```python
from build123d import *

# Parameters (mm, degrees)
SKETCH1_W           = 70
SKETCH1_H           = 132
BOSS_EXTRUDE1_DEPTH = 3
SKETCH2_R           = 1.6
SKETCH2_R_2         = 8
CUT_EXTRUDE1_DEPTH  = 75.76630257
CUT_EXTRUDE4_DEPTH  = 1


with BuildPart() as part:
    # Sketch1 → Boss-Extrude1 (new body)
    with BuildSketch(Plane.XY):
        Rectangle(SKETCH1_W, SKETCH1_H)
    extrude(amount=BOSS_EXTRUDE1_DEPTH)

    # Sketch2 → Cut-Extrude1 (cut, through all)
    with BuildSketch(Plane.XY.offset(3)):
        with Locations((0, 34)):
            Circle(SKETCH2_R)
        with Locations((12, 34)):
            Circle(SKETCH2_R)
        with Locations((6, 23.607695155)):
            Circle(SKETCH2_R)
        with Locations((-6, 23.607695155)):
            Circle(SKETCH2_R)
        with Locations((-12, 34)):
            Circle(SKETCH2_R)
        with Locations((-6, 44.392304845)):
            Circle(SKETCH2_R)
        with Locations((6, 44.392304845)):
            Circle(SKETCH2_R)
        with Locations((3, -43.897608135)):
            Circle(SKETCH2_R_2)
    extrude(amount=-CUT_EXTRUDE1_DEPTH, mode=Mode.SUBTRACT)

    # Sketch4 → Cut-Extrude4 (cut)
    # profile 1 of 3: a face of its own
    with BuildSketch(Plane.XY.offset(3)):
        with BuildLine():
            Line((12.435373561, 12.906743281), (-8.591322356, 12.79048604))
            add(Edge.make_bspline(
                [(-8.591322356, 12.79048604), (-8.704286114, 8.885776406), (-8.502594221, 1.79384743), (-8.325007333, -0.700797834)],
                knots=[3, 3, 3, 3, 4, 4, 4, 4], degree=3))
            add(Edge.make_bspline(
                [(-8.325007333, -0.700797834), (-7.927810309, -6.293112042), (-0.051557809, -7.493806409), (2.262018013, -2.357422472)],
                knots=[4, 4, 4, 4, 5, 5, 5, 5], degree=3))
            add(Edge.make_bspline(
                [(2.262018013, -2.357422472), (3.647515819, -6.937264415), (12.328667278, -6.654110228), (12.577245481, -0.371389262)],
                knots=[0, 0, 0, 0, 1, 1, 1, 1], degree=3))
            add(Edge.make_bspline(
                [(12.577245481, -0.371389262), (12.657220975, 1.669518266), (12.654067782, 9.68502366), (12.435373561, 12.906743281)],
                knots=[1, 1, 1, 1, 2, 2, 2, 2], degree=3))
        make_face()
        with BuildLine():
            Line((-4.326492155, 6.425883244), (-1.206711683, 6.455631236))
            add(Edge.make_bspline(
                [(-1.206711683, 6.455631236), (-1.074026475, 4.572236089), (-1.015280968, 2.842101206), (-2.419907538, 2.766134029)],
                knots=[1, 1, 1, 1, 2, 2, 2, 2], degree=3))
            add(Edge.make_bspline(
                [(-2.419907538, 2.766134029), (-3.973264085, 2.682447476), (-4.493703991, 3.948173451), (-4.326492155, 6.425883244)],
                knots=[2, 2, 2, 2, 3, 3, 3, 3], degree=3))
        make_face(mode=Mode.SUBTRACT)
        with BuildLine():
            Line((4.521297604, 6.43862815), (7.619481633, 6.437735553))
            add(Edge.make_bspline(
                [(7.619481633, 6.437735553), (7.754881729, 4.557137064), (7.590941128, 2.787865388), (6.186314558, 2.711898211)],
                knots=[1, 1, 1, 1, 2, 2, 2, 2], degree=3))
            add(Edge.make_bspline(
                [(6.186314558, 2.711898211), (4.635672899, 2.631008317), (4.351289109, 3.963633245), (4.521297604, 6.43862815)],
                knots=[2, 2, 2, 2, 3, 3, 3, 3], degree=3))
        make_face(mode=Mode.SUBTRACT)
    # profile 2 of 3: a face of its own
    with BuildSketch(Plane.XY.offset(3)):
        with BuildLine():
            add(Edge.make_bspline(
                [(3.36676789, -33.160113435), (9.417717715, -33.392835626), (13.445086014, -38.057518842), (13.529515019, -43.748190308), (13.613984909, -49.441617546), (9.14299869, -54.262705816), (3.092048865, -54.029983625)],
                knots=[2, 2, 2, 2, 3, 3, 3, 4, 4, 4, 4], degree=3))
            add(Edge.make_bspline(
                [(3.092048865, -54.029983625), (-2.961697619, -53.794546546), (-7.883326898, -49.978313982), (-8.018340697, -43.29333994)],
                knots=[0, 0, 0, 0, 1, 1, 1, 1], degree=3))
            add(Edge.make_bspline(
                [(-8.018340697, -43.29333994), (-8.133164977, -37.597606671), (-2.686937708, -32.927432129), (3.36676789, -33.160113435)],
                knots=[1, 1, 1, 1, 2, 2, 2, 2], degree=3))
        make_face()
    # profile 3 of 3: a face of its own
    with BuildSketch(Plane.XY.offset(3)):
        with BuildLine():
            add(Edge.make_bspline(
                [(-8.315009416, -8.062939687), (-4.406161921, -7.897447705), (8.068102589, -7.822629876), (12.839981265, -7.862087625)],
                knots=[11, 11, 11, 11, 12, 12, 12, 12], degree=3))
            add(Edge.make_bspline(
                [(12.839981265, -7.862087625), (12.861241838, -9.29508964), (12.9589587, -15.881387365), (12.980178387, -17.311633608)],
                knots=[0, 0, 0, 0, 1, 1, 1, 1], degree=3))
            add(Edge.make_bspline(
                [(12.980178387, -17.311633608), (11.763075071, -17.765199017), (8.114684439, -19.13687745), (7.383799305, -19.47848671)],
                knots=[1, 1, 1, 1, 2, 2, 2, 2], degree=3))
            add(Edge.make_bspline(
                [(7.383799305, -19.47848671), (9.108176948, -20.332188301), (12.314465086, -22.045945199), (12.935462432, -22.472239835)],
                knots=[2, 2, 2, 2, 3, 3, 3, 3], degree=3))
            add(Edge.make_bspline(
                [(12.935462432, -22.472239835), (12.97786092, -25.329976547), (12.909725475, -29.283635925), (12.92599799, -30.380433621)],
                knots=[3, 3, 3, 3, 4, 4, 4, 4], degree=3))
            add(Edge.make_bspline(
                [(12.92599799, -30.380433621), (7.795263549, -30.67706556), (-6.389215715, -30.667001608), (-7.858042781, -30.688793695)],
                knots=[4, 4, 4, 4, 5, 5, 5, 5], degree=3))
            add(Edge.make_bspline(
                [(-7.858042781, -30.688793695), (-8.0102064, -28.607228198), (-7.705115353, -24.647296875), (-7.841129113, -23.654261755)],
                knots=[5, 5, 5, 5, 6, 6, 6, 6], degree=3))
            add(Edge.make_bspline(
                [(-7.841129113, -23.654261755), (-4.784976738, -23.608919496), (1.083266322, -23.417113542), (2.673347405, -23.393522483)],
                knots=[6, 6, 6, 6, 7, 7, 7, 7], degree=3))
            add(Edge.make_bspline(
                [(2.673347405, -23.393522483), (-0.775407881, -21.686119301), (-3.737511671, -20.081751157), (-4.722867923, -19.434839155)],
                knots=[7, 7, 7, 7, 8, 8, 8, 8], degree=3))
            add(Edge.make_bspline(
                [(-4.722867923, -19.434839155), (-2.664517487, -18.089507553), (0.355778115, -15.627352279), (1.448315671, -14.952368219)],
                knots=[8, 8, 8, 8, 9, 9, 9, 9], degree=3))
            add(Edge.make_bspline(
                [(1.448315671, -14.952368219), (-3.198997245, -15.134329121), (-7.2306933, -15.194144924), (-8.333002543, -15.21049921)],
                knots=[9, 9, 9, 9, 10, 10, 10, 10], degree=3))
            add(Edge.make_bspline(
                [(-8.333002543, -15.21049921), (-8.355857659, -13.670022044), (-8.425935777, -8.946626939), (-8.315009416, -8.062939687)],
                knots=[10, 10, 10, 10, 11, 11, 11, 11], degree=3))
        make_face()
    extrude(amount=-CUT_EXTRUDE4_DEPTH, mode=Mode.SUBTRACT)


solid = part.part
```
Geometry: final body of the model. Coordinates: model frame, mm. A direction names the side the tool comes from. Round coordinates to 2 decimals unless told otherwise and drop trailing zeros. Order: outer loops, then holes, each group sorted by start corner. A loop starts at its lowest first (then second) coordinate and runs counter-clockwise, first axis right, second up. Notation, with made-up numbers: (35, -25.5) -> (68, -25.5) arc R23 ccw to (68, -4.5) -> close; hole circle Ø6 at (39.25, 38.5). An arc over 180 degrees is marked (long way). Use CSV: the item, a comma, the result in double quotes. Start each with the question number.
1) Draft query along X for faces 1 (the face through (-35, -1, 1)), 2 (the face through (-13.27, 33.03, 1.52)), 3 (the face through (0, -66, 1)). Return one class per face: +X half, -X half, draft (parallel to the pull), parting line (faces both ways), or undercut.
2) First-contact query: pin 1 Ø4 at (x, y) = (-28, -32) entering from -Z. Flat tip, straight axial feed; report the tip coordinate or a pass-through.
3) Section B-B (z = 1.15). State how many separate pieces and enclosed holes the cut face has, and give its area (3 significant figures).
4) Section A-A (y = 34). Return the cut outline in (x, z), and give its area (3 significant figures).
5) Set-up query: faces 4 (the face through (6, -36, 2)), 5 (the face through (6.86, 24.957, 1.521)). Return all of +Z, -Z, +X, -X, +Y, -Y with unobstructed straight access to the full face (end or side cutting, diameter ignored); none if empty.
6) Material intervals for line 1 along Y through (x, z) = (3, 0.55); line 2 along Y through (x, z) = (12, 1.75); line 3 along Y through (x, z) = (11, 2.65), sorted ascending. Write a range as from..to.
Returned:
1,face 1,"-X half"
1,face 2,"undercut"
1,face 3,"draft"
2,pin 1,"stops at z = 0"
3,separate pieces,"1"
3,enclosed holes,"8"
3,area,"8,980 mm²"
4,outline,"(-35, 0) -> (-13.6, 0) -> (-13.6, 3) -> (-35, 3) -> close; (-10.4, 0) -> (-1.6, 0) -> (-1.6, 3) -> (-10.4, 3) -> close; (1.6, 0) -> (10.4, 0) -> (10.4, 3) -> (1.6, 3) -> close; (13.6, 0) -> (35, 0) -> (35, 3) -> (13.6, 3) -> close"
4,area,"181 mm²"
5,face 4,"+Z"
5,face 5,"+Z, -Z"
6,line 1,"y = -66..-51.9, -35.9..66"
6,line 2,"y = -66..32.4, 35.6..66"
6,line 3,"y = -66..-50.69, -36.76..-30.47, -21.37..-18.06, -7.85..-4.03, 12.9..32.75, 35.25..66"
